Study the drawing (mm; zero at the part's minimum x, y, z) and answer. A direction names the side the tool comes from. Coordinates: 2 decimals unless noted, no trailing zeros. Order: outer loops, then holes, each group sorted by start corner. A loop starts at its lowest first (then second) coordinate and runs counter-clockwise, first axis right, second up. Notation, with made-up numbers: M -15.75,-11 L -6.75,-11 A22 ccw -6.75,3 Z; hole C -10,88 d8. An arc over 180 degrees is marked long. One line per item, written item: value. Start each with the question number.
Q1. The part is cut by section B-B on z = 40. Give the vertices of the cut face in (x, y).
Q2. The part is cut by section D-D on y = 69.5. Give the number of separate pieces and of enclosed holes in the cut face.
Q3. For the marked faces 1 and 2, determine the directions among +Z, -Z, +X, -X, +Y, -Y from which every point of the face is accessible in a straight line to the end or side of a thin tool.
Q4. The part is cut by section A-A on y = 40. Give the vertices of the cut face in (x, z).
Q5. Determine the mould class of the marked faces 3, 4, 5 and 6 for opening direction X: pulls with the +X half, pulls with the -X half, needs draft (parallel to the pull), parting line crosses it, or undercut.
Q6. Straight lines are drawn through the part: line 1 along Y through (x, z) = (15.25, 40); line 2 along X through (y, z) = (13.5, 26.5); line 3 along X through (y, z) = (4.5, 35) (1 decimal). For each, find the intervals that lie inside material, in ascending order. Write a range as [from, to].
Q7. The part is cut by section C-C on x = 8.5. Give the vertices of the cut face in (y, z).
Q8. Each of these flat-tipped pins is pushed along its axis until it touches: pin 1 Ø9 at (x, z) = (19, 39) entering from +Y; pin 2 Ø8 at (x, y) = (23.5, 41) entering from -Z; pin 3 Ø12 at (x, y) = (25.5, 14.5) entering from +Z (1 decimal); pin 4 Ø12 at (x, y) = (3, 68.5) entering from +Z. Where does it stop, or does it pass through?
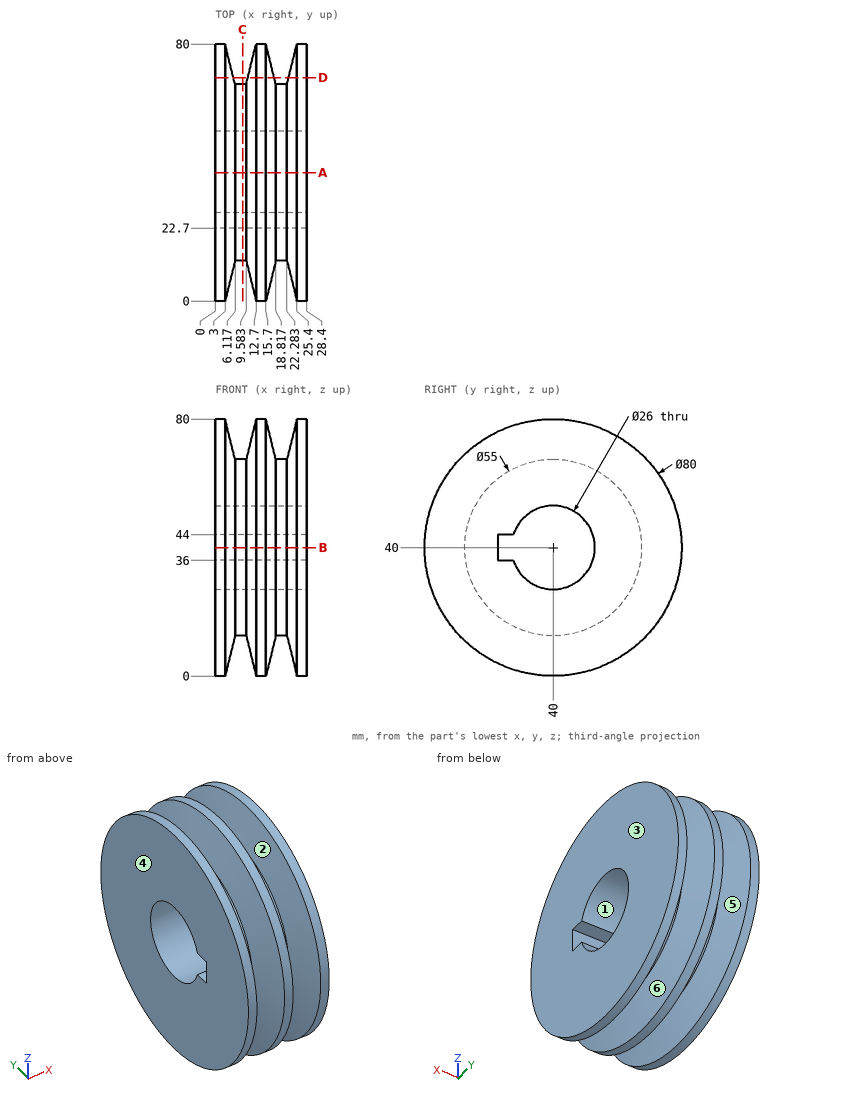
Output:
1. outline: M 0,0 L 3,0 L 6.12,12.5 L 9.58,12.5 L 12.7,0 L 15.7,0 L 18.82,12.5 L 22.28,12.5 L 25.4,0 L 28.4,0 L 28.4,22.7 L 0,22.7 Z; M 0,53 L 28.4,53 L 28.4,80 L 25.4,80 L 22.28,67.5 L 18.82,67.5 L 15.7,80 L 12.7,80 L 9.58,67.5 L 6.12,67.5 L 3,80 L 0,80 Z
2. separate pieces: 3
2. enclosed holes: 0
3. face 1: +X, -X
3. face 2: none
4. outline: M 0,0 L 3,0 L 6.12,12.5 L 9.58,12.5 L 12.7,0 L 15.7,0 L 18.82,12.5 L 22.28,12.5 L 25.4,0 L 28.4,0 L 28.4,27 L 0,27 Z; M 0,53 L 28.4,53 L 28.4,80 L 25.4,80 L 22.28,67.5 L 18.82,67.5 L 15.7,80 L 12.7,80 L 9.58,67.5 L 6.12,67.5 L 3,80 L 0,80 Z
5. face 3: pulls with the +X half
5. face 4: pulls with the -X half
5. face 5: undercut
5. face 6: undercut
6. line 1: y = [0, 22.7], [53, 80]
6. line 2: x = [0, 5.56], [10.14, 18.26], [22.84, 28.4]
6. line 3: x = [0, 4], [11.7, 16.7], [24.4, 28.4]
7. outline: C 40,40 d55; hole M 22.7,36 L 27.63,36 A13 ccw long 27.63,44 L 22.7,44 Z
8. pin 1: stops at y = 80
8. pin 2: stops at z = 0
8. pin 3: stops at z = 74.9
8. pin 4: stops at z = 73.07
